```python
from build123d import *

# Parameters (mm, degrees)
SKETCH1_W           = 38.1
SKETCH1_H           = 38.1
SKETCH1_R           = 2.286
SKETCH1_R_2         = 11.1125
BOSS_EXTRUDE1_DEPTH = 9.525


with BuildPart() as part:
    # Sketch1 → Boss-Extrude1 (new body)
    with BuildSketch(Plane(origin=(0, 0, 0), x_dir=(1, 0, 0), z_dir=(0, 1, 0))):
        Rectangle(SKETCH1_W, SKETCH1_H)
        with Locations((14.142135624, 14.142135624)):
            Circle(SKETCH1_R, mode=Mode.SUBTRACT)
        with Locations((14.142135624, -14.142135624)):
            Circle(SKETCH1_R, mode=Mode.SUBTRACT)
        with Locations((-14.142135624, -14.142135624)):
            Circle(SKETCH1_R, mode=Mode.SUBTRACT)
        with Locations((-14.142135624, 14.142135624)):
            Circle(SKETCH1_R, mode=Mode.SUBTRACT)
        Circle(SKETCH1_R_2, mode=Mode.SUBTRACT)
    extrude(amount=BOSS_EXTRUDE1_DEPTH)


solid = part.part
```
The model under review builds one solid part; all positions refer to its coordinate system, in mm. Round coordinates to 2 decimals unless told otherwise and drop trailing zeros. Loops run counter-clockwise (first coordinate to the right, second up) from the corner with the lowest first, then second, coordinate; pieces in that order, holes last. Notation, with made-up numbers: M 16.25,-34 L 44.25,-34 A28 ccw 44.25,5 Z; hole C 88,74.5 d11. An arc over 180 degrees is marked long. Answer as a JSON object with one key per item and string values.
(1) Take a section at B-B on x = 4.5. Give the boundary of the cut face in (y, z) (3 decimals), and give its area (3 significant figures).
Resolved:
{"outline": "M 0,-19.05 L 9.525,-19.05 L 9.525,-10.161 L 0,-10.161 Z; M 0,10.161 L 9.525,10.161 L 9.525,19.05 L 0,19.05 Z", "area": "169 mm²"}
(2) Take a section at D-D on z = -12.5. Give the boundary of the cut face in (x, y) (3 decimals), and give its area (3 significant figures).
Resolved:
{"outline": "M -19.05,0 L -15.732,0 L -15.732,9.525 L -19.05,9.525 Z; M -12.552,0 L 12.552,0 L 12.552,9.525 L -12.552,9.525 Z; M 15.732,0 L 19.05,0 L 19.05,9.525 L 15.732,9.525 Z", "area": "302 mm²"}
(3) Draft analysis for pull direction Z (two halves, no side actions). For faces 1 (the flat face through (19.05, 5, 0)), 2 (the cylindrical face through (12.46, 4.7, -15.69)), 3 (the flat face through (0, 5, 19.05)), state which applies: released by +Z, released by -Z, zero draft, split by the parting line, or undercut.
Resolved:
{"face 1": "zero draft", "face 2": "undercut", "face 3": "released by +Z"}
(4) Take a section at C-C on y = 1.5. Count the separate pieces of the cut face and the enclosed holes in it, and give its area (3 significant figures).
Resolved:
{"separate pieces": "1", "enclosed holes": "5", "area": "998 mm²"}
(5) Clearance check with flat-ended pins moving along their axes: P1, Ø4, axis at x = -14.14, z = 14.14, coming from the -Y side; P2, Ø10, axis at x = -7, z = -2, coming from the -Y side. State where each tip first meets the part, or that it passes through.
Resolved:
{"P1": "through", "P2": "y = 0"}
(6) To check wall thickness, follow line 1 along X through (y, z) = (5.5, 0); line 2 along X through (y, z) = (8.5, -14.5); line 3 along Z through (x, y) = (0.5, 8.75). State the ranges of each line that lie inside material, in increasing order.
Resolved:
{"line 1": "-19.05 to -11.11, 11.11 to 19.05", "line 2": "-19.05 to -16.4, -11.88 to 11.88, 16.4 to 19.05", "line 3": "-19.05 to -11.1, 11.1 to 19.05"}
